from build123d import *


# Not quite as in the source:
# - a fillet or chamfer that OpenCascade refuses, or shapes differently, is made with other operations: its cross-section is extruded or revolved along the edge and cut away or added


with BuildPart() as f1:
    # F0 (on Front) → F1 (revolve)
    with BuildSketch(Plane.XZ):
        Polygon((-22.5108576886, 12.7), (-41.5608576886, 12.7), (-41.5608576886, 9.525), (-22.5108576886, 7.9375), (-6.6358576886, 7.9375), (-6.6358576886, 12.7), (-19.3358576886, 12.7), (-19.3358576886, 15.875), (-22.5108576886, 15.875), align=None)
    revolve(axis=Axis((-22.7388739586, 0, 0), (-1, 0, 0)))

    # F2: chamfer of 0.508 on 6 edges, made by hand

    # F2_s1 → F2_t2 (revolve, cut)
    with BuildSketch(Plane.XZ):
        Polygon((-22.0028576886, 15.875), (-22.5108576886, 15.367), (-22.5108576886, 15.875), align=None)
    revolve(axis=Axis((-22.5108576886, 0, 0), (-1, 0, 0)), mode=Mode.SUBTRACT)

    # F2_s3 → F2_t4 (revolve, cut)
    with BuildSketch(Plane.XZ):
        Polygon((-19.3358576886, 15.367), (-19.8438576886, 15.875), (-19.3358576886, 15.875), align=None)
    revolve(axis=Axis((-19.3358576886, 0, 0), (-1, 0, 0)), mode=Mode.SUBTRACT)

    # F2_s5 → F2_t6 (revolve, cut)
    with BuildSketch(Plane.XZ):
        Polygon((-41.0528576886, 12.7), (-41.5608576886, 12.192), (-41.5608576886, 12.7), align=None)
    revolve(axis=Axis((-41.5608576886, 0, 0), (-1, 0, 0)), mode=Mode.SUBTRACT)

    # F2_s7 → F2_t8 (revolve, cut)
    with BuildSketch(Plane.XZ):
        Polygon((-6.6358576886, 12.192), (-7.1438576886, 12.7), (-6.6358576886, 12.7), align=None)
    revolve(axis=Axis((-6.6358576886, 0, 0), (-1, 0, 0)), mode=Mode.SUBTRACT)

    # F2_s9 → F2_t10 (revolve, cut)
    with BuildSketch(Plane.XZ):
        Polygon((-41.5608576886, 9.9924275038), (-41.0950447924, 9.4861822586), (-41.5608576886, 9.525), align=None)
    revolve(axis=Axis((-41.5608576886, 0, 0), (-1, 0, 0)), mode=Mode.SUBTRACT)

    # F2_s11 → F2_t12 (revolve, cut)
    with BuildSketch(Plane.XZ):
        Polygon((-7.1438576886, 7.9375), (-6.6358576886, 8.4455), (-6.6358576886, 7.9375), align=None)
    revolve(axis=Axis((-6.6358576886, 0, 0), (-1, 0, 0)), mode=Mode.SUBTRACT)


solid = f1.part
The listing builds one solid part. Answer for the finished solid, in the listing's coordinates (mm). A direction names the side the tool comes from. Round coordinates to 2 decimals unless told otherwise and drop trailing zeros. Loops run counter-clockwise (first coordinate to the right, second up) from the corner with the lowest first, then second, coordinate; pieces in that order, holes last. Notation, with made-up numbers: M 83.25,44 L 130.25,44 A23 ccw 130.25,60 Z; hole C -23.5,71.25 d5. An arc over 180 degrees is marked long. Return JSON: item names as keys, results as strings.
Q1. Each of these flat-tipped pins is pushed along its axis until it touches: pin 1 Ø8 at (x, y) = (-35.5, 10) entering from +Z; pin 2 Ø3 at (x, z) = (-26.5, -9.5) entering from -Y; pin 3 Ø4 at (x, z) = (-34.5, -9) entering from -Y; pin 4 Ø12.5 at (y, z) = (0, 0) entering from +X. Where does it stop, or does it pass through?
Results list:
{"pin 1": "stops at z = 11.19", "pin 2": "stops at y = -9.86", "pin 3": "stops at y = -10.6", "pin 4": "passes through"}
Q2. Find section D-D, the plane x = -30. Determine the outline of the cut face in (y, z).
Results list:
{"outline": "C 0,0 d25.4; hole C 0,0 d17.12"}
Q3. The mould has two halves that part along Y. Classify faces 1 (the face through (-31.91, -12.4, -2.75)), 2 (the face through (-14.72, -7.75, -1.72)), 3 (the face through (-41.561, 10, -2)): released by +Y, released by -Y, zero draft, split by the parting line, or undercut.
Results list:
{"face 1": "split by the parting line", "face 2": "undercut", "face 3": "zero draft"}
Q4. Find the intervals of material crossed by line 1 along Y through (x, z) = (-10.5, 0); line 2 along Y through (x, z) = (-19.5, 0); line 3 along X through (y, z) = (13.5, 7), in increasing order. Write a range as from..to.
Results list:
{"line 1": "y = -12.7..-7.94, 7.94..12.7", "line 2": "y = -15.53..-7.94, 7.94..15.53", "line 3": "x = -22.51..-19.34"}
Q5. Which of the six approach directions +Z, -Z, +X, -X, +Y, -Y give full straight-line access (tool end or side, diameter ignored) to faces 4 (the face through (-22.511, 11.5, -5.8)), 5 (the face through (-19.336, 11.5, 5.8)), 6 (the face through (-20.938, -15.497, -3.441))?
Results list:
{"face 4": "-X", "face 5": "+X", "face 6": "+X, -X"}
